Verification items for the finished model (mm, model axes). A direction names the side the tool comes from. Coordinates: 2 decimals unless noted, no trailing zeros. Loops run counter-clockwise (first coordinate to the right, second up) from the corner with the lowest first, then second, coordinate; pieces in that order, holes last. Notation, with made-up numbers: M 38,-29 L 67,-29 A17 cw 67,0 Z; hole C 35.25,29.25 d10. An arc over 180 degrees is marked long. Write item = value, one per line. Start each with the question number.
Autodesk Inventor part; units mm, degrees
ref_plane "YZ Plane" through (0, 0, 0) normal (1, 0, 0) x (0, 1, 0)
ref_plane "XZ Plane" through (0, 0, 0) normal (0, 1, 0) x (-1, 0, 0)
ref_plane "XY Plane" through (0, 0, 0) normal (0, 0, 1) x (1, 0, 0)
sketch "Sketch_1" plane through (0, 0, 0) normal (0, 0, 1) x (1, 0, 0)
  line L0 (0, 0) -> (-5, 0)
  line L1 (-5, 0) -> (-5, 2)
  line L2 (-5, 2) -> (-4, 3)
  line L3 (-4, 3) -> (0.5, 3)
  line L4 (0.5, 3) -> (0.5, 0)
  line L5 (0.5, 0) -> (-5, 0)
revolve "Revolution1" add sketch "Sketch_1" angle 360 about axis through (0, 0, 0) along (1, 0, 0)
sketch "Sketch_2" plane through (0, 0, 0) normal (0, 0, 1) x (1, 0, 0)
  line L0 (7, 0) -> (0, 0)
  line L1 (0, 0) -> (0, 1)
  line L2 (0, 1) -> (5, 1)
  line L3 (5, 1) -> (7, 0.4641)
  line L4 (7, 0.4641) -> (7, 0)
  line L5 (7, 0) -> (0, 0)
revolve "Revolution2" add sketch "Sketch_2" angle 360 about axis through (7, 0, 0) along (1, 0, 0)
sketch "Sketch_13" plane through (0, 0, 0) normal (0, 0, 1) x (1, 0, 0)
  line L0 (50, 0) -> (-50, 0)
  line L1 (0, 6) -> (0, 1.15)
  arc A0 (0, 1.15) -> (0.2, 0.95) centre (0.2, 1.15) ccw
  line L2 (0.2, 0.95) -> (0.3677, 0.95)
  arc A1 (0.3677, 0.95) -> (0.5, 1) centre (0.3677, 1.15) ccw
  line L3 (0.5, 1) -> (0.5, 6)
  line L4 (0.5, 6) -> (0, 6)
revolve "Revolution3" cut sketch "Sketch_13" angle 360 about axis through (50, 0, 0) along (1, 0, 0)
properties part number "SFPSA6-P2-L5-B5"
Q1. Gauge pin test, flat ends, axial feed: pin 1 (1 mm diameter, centred on x = 1.5, y = -0.5, fed in from +Z); pin 2 (1.5 mm diameter, centred on x = -3, z = -2, fed in from +Y). Record the tip position at first contact, or that the pin passes through.
Q2. Set-up check for faces 1 (the face through (-2, -3, 0)), 2 (the face through (0, 1.3, 0)): record each of +Z, -Z, +X, -X, +Y, -Y from which the full face is reachable in a straight line by a thin tool's end or side.
Q3. Sectioned sample at A-A on y = 0. Record the cut outline in (x, z), plus the area to 3 significant figures.
Q4. Mould release check, pull along X, two halves, no side actions. Record for faces 3 (the face through (-5, 0, 0)), 4 (the face through (6.208, 0.645, -0.203)), 5 (the face through (3, 0, -1)): +X half, -X half, draft (parallel to the pull), parting line (faces both ways), or undercut.
Q5. Sectioned sample at C-C on x = 4.5. Record the cut outline in (y, z), plus the area to 3 significant figures.
Q6. Sectioned sample at D-D on x = 6. Record the cut outline in (y, z), plus the area to 3 significant figures.
Q7. Scan lines: L1, parallel to X at y = -1.5, z = 1.25; L2, parallel to Z at x = 3, y = 0.1; L3, parallel to Z at x = -1.25, y = 1.9. Record each from-to range of solid material in increasing order. Write a range as [from, to].
Solutions:
q1.pin_1 = 1
q1.pin_2 = 2.73
q2.face_1 = +X, -X
q2.face_2 = +X
q3.outline = M -5,-2 L -4,-3 L 0,-3 L 0,-1.15 A0.2 cw 0.2,-0.95 L 0.37,-0.95 A0.2 cw 0.5,-1 L 5,-1 L 7,-0.46 L 7,0.46 L 5,1 L 0.5,1 A0.2 cw 0.37,0.95 L 0.2,0.95 A0.2 cw 0,1.15 L 0,3 L -4,3 L -5,2 Z
q3.area = 41.9 mm²
q4.face_3 = -X half
q4.face_4 = +X half
q4.face_5 = draft
q5.outline = C 0,0 d2
q5.area = 3.14 mm²
q6.outline = C 0,0 d1.46
q6.area = 1.68 mm²
q7.L1 = [-5, 0]
q7.L2 = [-0.99, 0.99]
q7.L3 = [-2.32, 2.32]
